```python
from build123d import *

# Parameters (mm, degrees)
F1_DEPTH = 4.5
F2_R     = 2.99999
F3_R     = 3.99999


# Not quite as in the source:
# - a fillet or chamfer is up to 0.001 mm smaller than in the source, because OpenCascade refuses the exact size


with BuildPart() as f1:
    # F0 (on Top) → F1 (new body)
    with BuildSketch(Plane.XY):
        Polygon((10.5, 3), (10.5, 0), (11.5, 0), (11.5, 4), (-11.5, 4), (-11.5, 0), (-10.5, 0), (-10.5, 3), align=None)
    extrude(amount=F1_DEPTH)

    # F2 (radius 3 in the source; OpenCascade refuses exactly that, so slightly less here)
    f2_edges = [f1.edges().sort_by_distance(p)[0] for p in [
        (10.5, 3, 2.25),
        (-10.5, 3, 2.25),
    ]]
    fillet(f2_edges, radius=F2_R)

    # F3 (radius 4 in the source; OpenCascade refuses exactly that, so slightly less here)
    f3_edges = [f1.edges().sort_by_distance(p)[0] for p in [
        (-11.5, 4, 2.25),
        (11.5, 4, 2.25),
    ]]
    fillet(f3_edges, radius=F3_R)


solid = f1.part
```
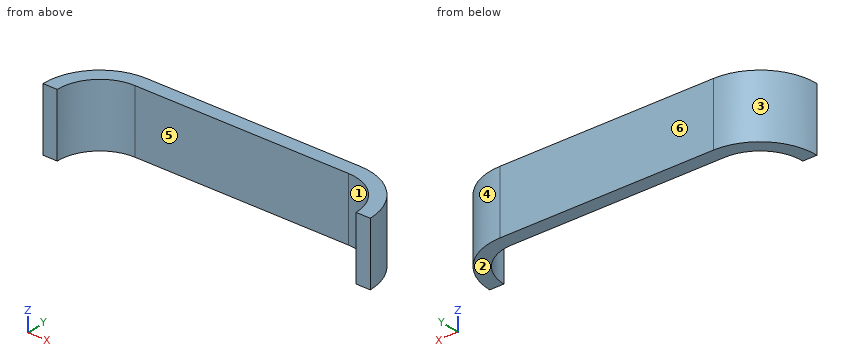
The model under review builds one solid part; all positions refer to its coordinate system, in mm. Face numbers are marked on the shaded views. A direction names the side the tool comes from. Round coordinates to 2 decimals unless told otherwise and drop trailing zeros. Order: outer loops, then holes, each group sorted by start corner. A loop starts at its lowest first (then second) coordinate and runs counter-clockwise, first axis right, second up. Notation, with made-up numbers: (13.5, 43.5) -> (70.5, 43.5) arc R37 cw to (70.5, 79.5) -> close; hole circle Ø8 at (87, 40.5). An arc over 180 degrees is marked (long way). One line per item, written item: value. Start each with the question number.
Q1. Wall thickness on line 1 (Y direction, x = 0.75, z = 3.9); line 2 (X direction, y = 2.7, z = 0.4); line 3 (X direction, y = 2.35, z = 4): over which ranges is each line inside the solid? List them lowest first.
Q2. Take a section at A-A (y = 2.65). Write out the cut boundary in (x, z), and give its area (3 significant figures).
Q3. Mouldability with a two-part tool opening along X and no side actions: class the marked faces 3, 4, 5 and 6 as released by +X, released by -X, zero draft, split by the parting line, or undercut.
Q4. Clearance check with flat-ended pins moving along their axes: pin 1 Ø1.5 at (y, z) = (3.5, 3.5) entering from +X; pin 2 Ø2 at (x, y) = (0, 2.5) entering from +Z. State where each tip first meets the part, or that it passes through.
Q5. Take a section at D-D (y = 1.25). Write out the cut boundary in (x, z).
Q6. Take a section at C-C (x = 2). Write out the cut boundary in (y, z), and give its area (3 significant figures).
Q7. Machinability: for the marked faces 1 and 2, which of the approach directions +Z, -Z, +X, -X, +Y, -Y give a long, thin tool a straight path to every point of the face, cutting with its end or side? Answer none if there is none.
Reported:
1. line 1: y = 3 to 4
1. line 2: x = -10.45 to -8.81, 8.81 to 10.45
1. line 3: x = -10.74 to -9.36, 9.36 to 10.74
2. outline: (-10.5, 0) -> (-8.91, 0) -> (-8.91, 4.5) -> (-10.5, 4.5) -> close; (8.91, 0) -> (10.5, 0) -> (10.5, 4.5) -> (8.91, 4.5) -> close
2. area: 14.3 mm2
3. face 3: released by -X
3. face 4: released by +X
3. face 5: undercut
3. face 6: zero draft
4. pin 1: stops at x = 10.4
4. pin 2: stops at z = 4.5
5. outline: (-11.3, 0) -> (-10.23, 0) -> (-10.23, 4.5) -> (-11.3, 4.5) -> close; (10.23, 0) -> (11.3, 0) -> (11.3, 4.5) -> (10.23, 4.5) -> close
6. outline: (3, 0) -> (4, 0) -> (4, 4.5) -> (3, 4.5) -> close
6. area: 4.50 mm2
7. face 1: +Z, -Z, -Y
7. face 2: -Z, +X, -X, +Y, -Y
